```python
from build123d import *

# Parameters (mm, degrees)
BOSS_EXTRUDE2_DEPTH  = 3.175
SKETCH6_W            = 19.05
SKETCH6_H            = 3.175
CUT_EXTRUDE5_DEPTH   = 3.175
LPATTERN1_COUNT      = 2
LPATTERN1_PITCH      = 114.3
LPATTERN1_COUNT_DIR2 = 2
LPATTERN1_PITCH_DIR2 = 44.45
SKETCH7_R            = 12.7
CUT_EXTRUDE6_DEPTH   = 3.175
LPATTERN2_COUNT      = 2
LPATTERN2_PITCH      = 50.8
LPATTERN2_COL_COUNT  = 2
LPATTERN2_COL_PITCH  = 50.8


with BuildPart() as part:
    # Sketch1 → Boss-Extrude2 (new body)
    with BuildSketch(Plane(origin=(0, 0, 0), x_dir=(1, 0, 0), z_dir=(0, 1, 0))):
        Polygon((24.645444356, 45.246601981), (-63.5, 36.321593844), (-88.9, 34.035796922), (-88.9, 30.860796922), (-114.3, 30.860796922), (-114.3, -30.860796922), (-88.9, -30.860796922), (-88.9, -34.035796922), (-63.5, -36.321593844), (24.645444356, -45.246601981), (57.256759974, -45.246601981), (57.256759974, -48.548601981), (63.5, -49.18075), (63.5, 49.18075), (57.256759974, 48.548601981), (57.256759974, 45.246601981), align=None)
    extrude(amount=BOSS_EXTRUDE2_DEPTH)

    # Sketch6 → Cut-Extrude5 (cut)
    with BuildSketch(Plane(origin=(0, 3.175, 0), x_dir=(1, 0, 0), z_dir=(0, 1, 0))):
        with Locations((-79.375, 22.923296922)):
            Rectangle(SKETCH6_W, SKETCH6_H)
    cut_extrude5 = extrude(amount=-CUT_EXTRUDE5_DEPTH, mode=Mode.SUBTRACT)

    # LPattern1: Cut-Extrude5 2 × 2
    with Locations(*[(i * LPATTERN1_PITCH, 0, j * LPATTERN1_PITCH_DIR2) for i in range(LPATTERN1_COUNT) for j in range(LPATTERN1_COUNT_DIR2) if (i, j) != (0, 0)]):
        add(cut_extrude5, mode=Mode.SUBTRACT)

    # Sketch7 → Cut-Extrude6 (cut)
    with BuildSketch(Plane(origin=(0, 3.175, 0), x_dir=(1, 0, 0), z_dir=(0, 1, 0))):
        with Locations((-25.4, 0)):
            Circle(SKETCH7_R)
    cut_extrude6 = extrude(amount=-CUT_EXTRUDE6_DEPTH, mode=Mode.SUBTRACT)

    # LPattern2: Cut-Extrude6 ×2
    with Locations(*[(-i * LPATTERN2_PITCH, 0, 0) for i in range(1, LPATTERN2_COUNT)]):
        add(cut_extrude6, mode=Mode.SUBTRACT)

    # LPattern2 col: Cut-Extrude6 ×2
    with Locations(*[(i * LPATTERN2_COL_PITCH, 0, 0) for i in range(1, LPATTERN2_COL_COUNT)]):
        add(cut_extrude6, mode=Mode.SUBTRACT)


solid = part.part
```
For this review, take the finished solid that the model builds, in its own axes (mm). A direction names the side the tool comes from. Round coordinates to 2 decimals unless told otherwise and drop trailing zeros. Write each loop counter-clockwise with the first axis right and the second up, starting at its lowest first coordinate (ties: lowest second). Pieces come first, ordered by that corner, then holes. Notation, with made-up numbers: (59.25, 69) - (104.25, 69) arc R16 ccw to (104.25, 98) - close; hole circle Ø4 at (66, 28.5). An arc over 180 degrees is marked (long way). Answer as a JSON object with one key per item and string values.
1. We need section D-D on x = -29. Give the boundary of the cut face in (y, z) (3 decimals).
Response values:
{"outline": "(0, -39.815) - (3.175, -39.815) - (3.175, -12.179) - (0, -12.179) - close; (0, 12.179) - (3.175, 12.179) - (3.175, 39.815) - (0, 39.815) - close"}
2. We need section A-A on z = 0. Give the boundary of the cut face in (x, y) (3 decimals).
Response values:
{"outline": "(-114.3, 0) - (-88.9, 0) - (-88.9, 3.175) - (-114.3, 3.175) - close; (-63.5, 0) - (-38.1, 0) - (-38.1, 3.175) - (-63.5, 3.175) - close; (-12.7, 0) - (12.7, 0) - (12.7, 3.175) - (-12.7, 3.175) - close; (38.1, 0) - (63.5, 0) - (63.5, 3.175) - (38.1, 3.175) - close"}
3. To check wall thickness, follow line 1 along X through (y, z) = (0.9, 0); line 2 along Z through (x, y) = (-76.2, 2.15); line 3 along X through (y, z) = (1.15, 8.5). State the ranges of each line that lie inside material, in increasing order.
Response values:
{"line 1": "x = -114.3 to -88.9, -63.5 to -38.1, -12.7 to 12.7, 38.1 to 63.5", "line 2": "z = -35.18 to -24.51, -21.34 to -12.7, 12.7 to 19.94, 23.11 to 35.18", "line 3": "x = -114.3 to -85.64, -66.76 to -34.84, -15.96 to 15.96, 34.84 to 63.5"}
4. We need section C-C on y = 1.55. Count the separate pieces of the cut face and the enclosed holes in it, then the cut area to 3 significant figures.
Response values:
{"separate pieces": "1", "enclosed holes": "7", "area": "12,300 mm2"}
5. Draft analysis for pull direction Z (two halves, no side actions). For faces 6 (the face through (-101, 2, -30.861)), 7 (the face through (57.257, 2, 47)), 8 (the face through (-88.9, 2, -23)), state which applies: +Z half, -Z half, draft (parallel to the pull), parting line (faces both ways), or undercut.
Response values:
{"face 6": "-Z half", "face 7": "draft", "face 8": "undercut"}
6. Tool access review of faces 1 (the face through (63.5, 2, 1)), 2 (the face through (-88.9, 2, -32)), 3 (the face through (44.45, 2, 22)), 4 (the face through (-88.9, 2, 32)), 5 (the face through (-114.3, 2, 0)): name each direction out of +Z, -Z, +X, -X, +Y, -Y from which nothing blocks a thin tool from reaching the whole face with its end or side.
Response values:
{"face 1": "+Z, -Z, +X, +Y, -Y", "face 2": "-Z, -X, +Y, -Y", "face 3": "+Y, -Y", "face 4": "+Z, -X, +Y, -Y", "face 5": "+Z, -Z, -X, +Y, -Y"}
7. For pin 1 Ø10 at (x, z) = (-44.5, 20.5) entering from -Y; pin 2 Ø1 at (y, z) = (1, 32.5) entering from -X; pin 3 Ø1 at (x, y) = (-79.5, 1.5) entering from +Z; pin 4 Ø1.6 at (x, y) = (-83.5, 1.5) entering from -Z, all flat-tipped, find the tip position at first contact; note any pin that passes through.
Response values:
{"pin 1": "stops at y = 0", "pin 2": "stops at x = -88.9", "pin 3": "stops at z = 34.93", "pin 4": "stops at z = -34.59"}
8. We need section B-B on x = -85. Give the boundary of the cut face in (y, z) (3 decimals), then the cut area to 3 significant figures.
Response values:
{"outline": "(0, -34.387) - (3.175, -34.387) - (3.175, -24.511) - (0, -24.511) - close; (0, -21.336) - (3.175, -21.336) - (3.175, -9.157) - (0, -9.157) - close; (0, 9.157) - (3.175, 9.157) - (3.175, 19.939) - (0, 19.939) - close; (0, 23.114) - (3.175, 23.114) - (3.175, 34.387) - (0, 34.387) - close", "area": "140 mm2"}
